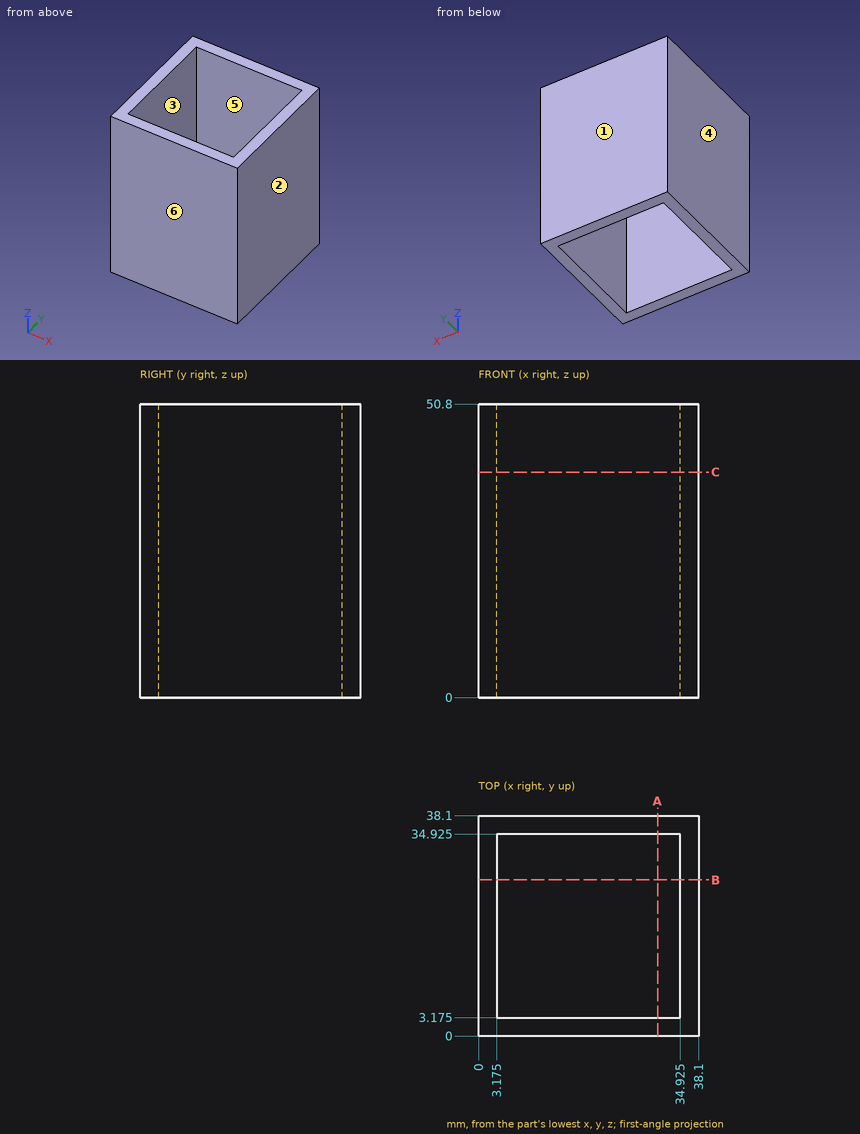
Job drawing, mm, ordinate dimensions from the low corner. One solid piece. A direction names the side the tool comes from. Coordinates: 2 decimals unless noted, no trailing zeros. Loops run counter-clockwise (first coordinate to the right, second up) from the corner with the lowest first, then second, coordinate; pieces in that order, holes last. Notation, with made-up numbers: (47.5, -15.5) -> (74.5, -15.5) arc R13 ccw to (74.5, 2.5) -> close; hole circle Ø2 at (-23, -7.75). An arc over 180 degrees is marked (long way). One line per item, written item: value.
1. Pull direction X, two halves, no side cores. Call the marked faces 1, 2, 3 and 4: pulls with the +X half, pulls with the -X half, needs draft (parallel to the pull), parting line crosses it, or undercut.
Answers:
face 1: needs draft
face 2: pulls with the +X half
face 3: undercut
face 4: pulls with the -X half
2. Slice it at C-C on z = 39. Write the cut outline in (x, y) (3 decimals).
Answers:
outline: (0, 0) -> (38.1, 0) -> (38.1, 38.1) -> (0, 38.1) -> close; hole (3.175, 3.175) -> (34.925, 3.175) -> (34.925, 34.925) -> (3.175, 34.925) -> close
3. Which spindle directions (+Z, -Z, +X, -X, +Y, -Y) get a long thin tool onto all of the face, cutting with end or side? Do the marked faces 5 and 6. Say none if no direction does.
Answers:
face 5: +Z, -Z
face 6: +Z, -Z, +X, -X, -Y
4. Drill centre line: line 1 (X direction, y = 9, z = 8) (3 decimals). Where is it in solid material? Low to high. Write a range as [from, to].
Answers:
line 1: x = [0, 3.175], [34.925, 38.1]
5. Slice it at A-A on x = 31. Write the cut outline in (y, z) (3 decimals), and give its area (3 significant figures).
Answers:
outline: (0, 0) -> (3.175, 0) -> (3.175, 50.8) -> (0, 50.8) -> close; (34.925, 0) -> (38.1, 0) -> (38.1, 50.8) -> (34.925, 50.8) -> close
area: 323 mm^2
